Source: CAD feature listing. Evaluate the final solid. Frame: model axes, mm. A direction names the side the tool comes from. Give positions to 0.01 mm unless a question says otherwise; leave off trailing zeros. Order: outer loops, then holes, each group sorted by start corner. A loop starts at its lowest first (then second) coordinate and runs counter-clockwise, first axis right, second up. Notation, with made-up numbers: (11.25, 87) -> (35.25, 87) arc R25 cw to (35.25, 102) -> close; hole circle Ø6 at (61.25, 84.5). An arc over 180 degrees is marked (long way). Use one line per item in the form item = value. Start each with the question number.
from build123d import *

# Parameters (mm, degrees)
CUT_EXTRUDE10_DEPTH = 1.48828125


with BuildPart() as part:
    # Sketch22 → Revolve1 (revolve)
    with BuildSketch(Plane(origin=(0, 0, 0), x_dir=(0, 0, -1), z_dir=(1, 0, 0)), mode=Mode.PRIVATE) as revolve1_sk:
        Polygon((-5.952759232, 0), (-5.952759232, 1.9304), (-5.614839074, 2.413), (5.656480087, 2.413), (6.747240768, 1.322239319), (5.952759232, 0), align=None)
    revolve(revolve1_sk.sketch.rotate(Axis((0, 0, -5.952759232), (0, 0, -1)), 180), axis=Axis((0, 0, -5.952759232), (0, 0, -1)))

    # Sketch23 → Cut-Extrude10 (cut)
    with BuildSketch(Plane.XY.offset(5.952759232)):
        Polygon((0, 1.374815329), (-1.190625, 0.687407664), (-1.190625, -0.687407664), (0, -1.374815329), (1.190625, -0.687407664), (1.190625, 0.687407664), align=None)
    extrude(amount=-CUT_EXTRUDE10_DEPTH, mode=Mode.SUBTRACT)

    # Cut-Extrude11 cone 1 section (on through the dimple's axis) → Cut-Extrude11 (revolve, cut)
    with BuildSketch(Plane(origin=(0, 0, 5.952759232), x_dir=(0, -1, 0), z_dir=(1, 0, 0))):
        Polygon((0, 0), (1.374815329, 0), (0, 1.374815329), align=None)
    revolve(axis=Axis((0, 0, 5.952759232), (0, 0, -1)), mode=Mode.SUBTRACT)

    # Cut-Extrude12 cone 1 section (on through the dimple's axis) → Cut-Extrude12 (revolve, cut)
    with BuildSketch(Plane(origin=(0, 0, 4.464477982), x_dir=(0, -1, 0), z_dir=(1, 0, 0))):
        Polygon((0, 0), (1.190625, 0), (0, 0.687407664), align=None)
    revolve(axis=Axis((0, 0, 4.464477982), (0, 0, -1)), mode=Mode.SUBTRACT)


solid = part.part
1) Pin query (flat end, axial travel): pin 1 (1 mm diameter, centred on x = 0, y = 1.5, fed in from -Z); pin 2 (1 mm diameter, centred on y = 1, z = 4.5, fed in from +X); pin 3 (1.5 mm diameter, centred on x = -1.5, z = -4.5, fed in from -Y). Return the tip coordinate at first contact, or that it passes through.
2) Cut plane A-A, the plane z = -1. Return the cut outline in (x, y), plus the area to 3 significant figures.
3) Material intervals for probe 1 along X at (y, z) = (-0.6, 4.75); probe 2 along Y at (x, z) = (2.15, -1.75); probe 3 along Y at (x, z) = (-0.25, -3.25), sorted ascending.
4) Draft query along Y for faces 1 (the face through (1.468, 1.915, -0.1)), 2 (the face through (-0.6, -1.03, 5.22)), 3 (the face through (1.3, 0.8, 5.953)). Return one class per face: +Y half, -Y half, draft (parallel to the pull), parting line (faces both ways), or undercut.
5) Reachability of faces 4 (the face through (0.6, 1.03, 5.22)), 5 (the face through (-0.06, -0.2, -6.08)) from +Z, -Z, +X, -X, +Y, -Y: full face, straight path, thin tool, end or side. Return the list, or none.
Output values:
q1.pin_1 = -6.75
q1.pin_2 = 2.36
q1.pin_3 = -2.29
q2.outline = circle Ø4.83 at (0, 0)
q2.area = 18.3 mm^2
q3.probe_1 = -2.34 to -1.19, 1.19 to 2.34
q3.probe_2 = -1.1 to 1.1
q3.probe_3 = -2.4 to 2.4
q4.face_1 = parting line
q4.face_2 = undercut
q4.face_3 = draft
q5.face_4 = +Z
q5.face_5 = -Z
